The figure shows three views and two pictorial views of one solid part (mm, origin at its lowest corner). Answer the questions. A direction names the side the tool comes from. Coordinates: 2 decimals unless noted, no trailing zeros. Loops run counter-clockwise (first coordinate to the right, second up) from the corner with the lowest first, then second, coordinate; pieces in that order, holes last. Notation, with made-up numbers: M 43.5,82 L 90.5,82 A32 ccw 90.5,109 Z; hole C 71,13.25 d9. An arc over 180 degrees is marked long. Answer as a JSON object with one key per item and string values. Group by question number.
1. A cutting plane is placed at A-A on y = 8. Give the vertices of the cut face in (x, z), and give its area (3 significant figures).
2. Straight lines are drawn through the part: L1, parallel to X at y = 15.5, z = 90.5; L2, parallel to Z at x = 98.5, y = 34.5; L3, parallel to Y at x = 38, z = 19. For each, find the intervals that lie inside material, in ascending order.
3. A cutting plane is placed at B-B on y = 36.5. Give the vertices of the cut face in (x, z), and give its area (3 significant figures).
4. A cutting plane is placed at C-C on x = 94. Give the vertices of the cut face in (y, z), and give its area (3 significant figures).
5. Determine the mould class of the marked faces 3, 4 and 5 for opening direction Z: released by +Z, released by -Z, zero draft, split by the parting line, or undercut.
6. A cutting plane is placed at D-D on z = 48. Give the vertices of the cut face in (x, y).
7. Given pin 1 (25 mm diameter, centred on x = 81.5, z = 135, fed in from +Y), flat-ended and moving along its own axis, determine where the tip first touches the part or whether it passes through.
8. For the marked faces 1 and 2, determine the directions among +Z, -Z, +X, -X, +Y, -Y from which every point of the face is accessible in a straight line to the end or side of a thin tool.
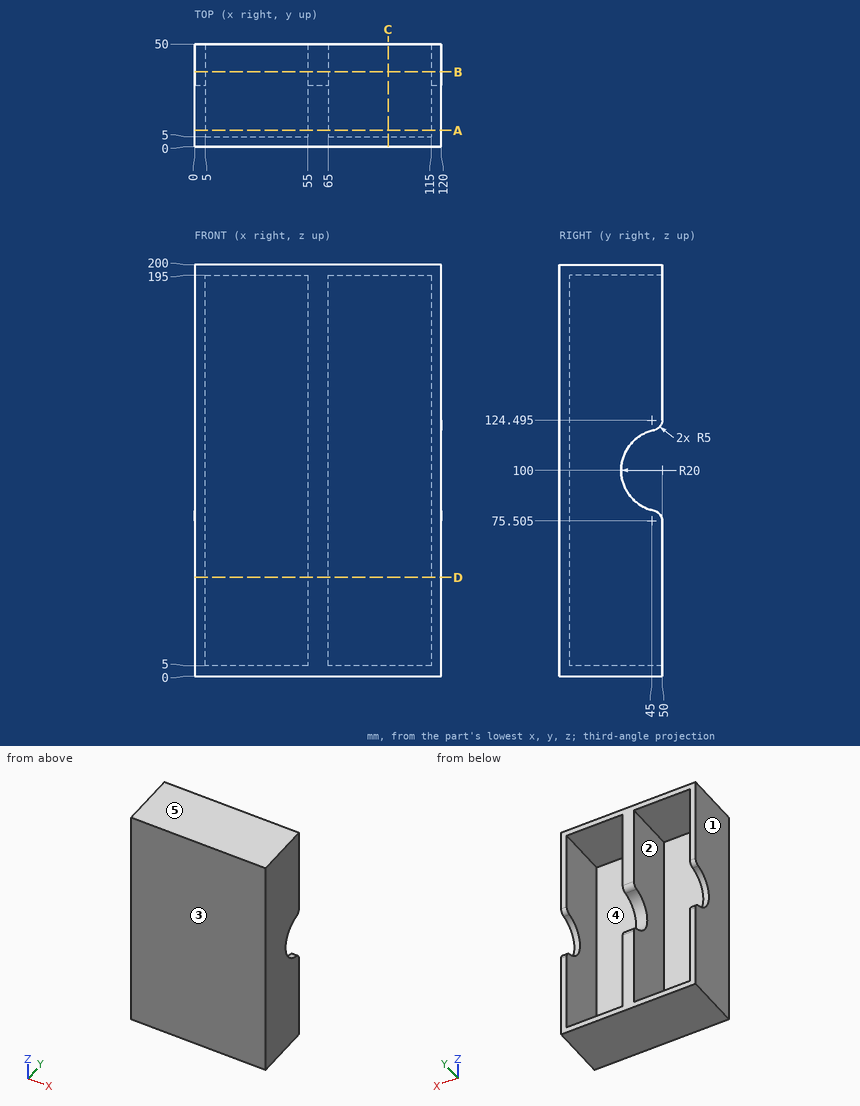
From the geometry:
{
 "1": {"outline": "M 0,0 L 120,0 L 120,200 L 0,200 Z; hole M 5,5 L 55,5 L 55,195 L 5,195 Z; hole M 65,5 L 115,5 L 115,195 L 65,195 Z", "area": "5,000 mm²"},
 "2": {"L1": "x = 0 to 5, 55 to 65, 115 to 120", "L2": "z = 0 to 5, 195 to 200", "L3": "y = 0 to 5"},
 "3": {"outline": "M 0,0 L 120,0 L 120,85.24 L 115,85.24 L 115,5 L 65,5 L 65,85.24 L 55,85.24 L 55,5 L 5,5 L 5,85.24 L 0,85.24 Z; M 0,114.76 L 5,114.76 L 5,195 L 55,195 L 55,114.76 L 65,114.76 L 65,195 L 115,195 L 115,114.76 L 120,114.76 L 120,200 L 0,200 Z", "area": "4,410 mm²"},
 "4": {"outline": "M 0,0 L 50,0 L 50,5 L 5,5 L 5,195 L 50,195 L 50,200 L 0,200 Z", "area": "1,450 mm²"},
 "5": {"face 3": "zero draft", "face 4": "undercut", "face 5": "released by +Z"},
 "6": {"outline": "M 0,0 L 120,0 L 120,50 L 115,50 L 115,5 L 65,5 L 65,50 L 55,50 L 55,5 L 5,5 L 5,50 L 0,50 Z"},
 "7": {"pin 1": "stops at y = 5"},
 "8": {"face 1": "+Z, -Z, -X, +Y, -Y", "face 2": "+Y"}
}
